Can you work these out from the model? Positions are in its coordinate system, mm. Face numbers are marked on the shaded views. A direction names the side the tool comes from. Coordinates: 2 decimals unless noted, no trailing zeros. Write each loop counter-clockwise with the first axis right and the second up, starting at its lowest first coordinate (ties: lowest second). Pieces come first, ordered by that corner, then holes.
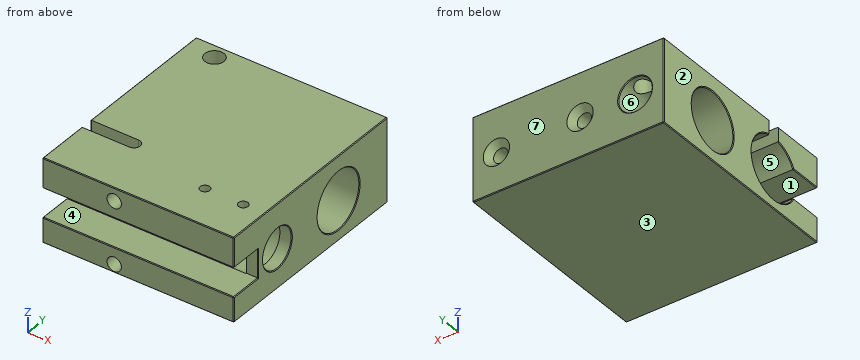
```python
from build123d import *

# Parameters (mm, degrees)
ESQUISSE1_W                   = 80
ESQUISSE1_H                   = 88
BASE_EXTRUSION_DEPTH          = 35
ESQUISSE4_R                   = 12
BOSS_EXTRU_2_DEPTH            = 80
ESQUISSE5_R                   = 12
ENL_V_MAT_EXTRU_1_DEPTH       = 145
ESQUISSE6_W                   = 12
ESQUISSE6_H                   = 14
ENL_V_MAT_EXTRU_2_DEPTH       = 145
ESQUISSE12_R                  = 12.75
ENL_V_MAT_EXTRU_4_DEPTH       = 75
ESQUISSE13_R                  = 8.25
ENL_V_MAT_EXTRU_5_DEPTH       = 94.733665244
ESQUISSE17_W                  = 20
ESQUISSE17_H                  = 5.2
ENL_V_MAT_EXTRU_9_DEPTH       = 10
ESQUISSE18_R                  = 2.6
ENL_V_MAT_EXTRU_10_DEPTH      = 10
ESQUISSE20_R                  = 2.25
ENL_V_MAT_EXTRU_12_DEPTH      = 14
ESQUISSE21_R                  = 3
ENL_V_MAT_EXTRU_13_DEPTH      = 10
CHANFREIN9_SIZE               = 1.154700538
CHANFREIN9_SIZE2              = 2
CHANFREIN20_SIZE              = 1.154700538
CHANFREIN20_SIZE2             = 2
ESQUISSE22_R                  = 2
ENL_V_MAT_EXTRU_15_DEPTH      = 5.5
ESQUISSE24_R                  = 7
ENL_V_MAT_EXTRU_23_DEPTH      = 25
ENL_V_MAT_EXTRU_24_REACH      = 71
ENL_V_MAT_EXTRU_24_END_RADIUS = 7
ESQUISSE25_R                  = 4
ESQUISSE26_R                  = 2.5
ENL_V_MAT_EXTRU_25_DEPTH      = 15
ESQUISSE28_R                  = 3
ENL_V_MAT_EXTRU_26_DEPTH      = 12
CHANFREIN27_SIZE              = 2.5
CHANFREIN29_SIZE              = 0.3


with BuildPart() as part:
    # Esquisse1 → Base-Extrusion (new body)
    with BuildSketch(Plane.XY):
        Rectangle(ESQUISSE1_W, ESQUISSE1_H)
    extrude(amount=BASE_EXTRUSION_DEPTH)

    # Esquisse4 → Boss.-Extru.2 (add, through all)
    with BuildSketch(Plane.ZY.offset(40)):
        with Locations((16.5, 16)):
            Circle(ESQUISSE4_R)
    extrude(amount=-BOSS_EXTRU_2_DEPTH)

    # Esquisse5 → Enlèv. mat.-Extru.1 (cut)
    with BuildSketch(Plane.ZY.offset(40)):
        with Locations((16.5, 16)):
            Circle(ESQUISSE5_R)
    extrude(amount=-ENL_V_MAT_EXTRU_1_DEPTH, mode=Mode.SUBTRACT)

    # Esquisse6 → Enlèv. mat.-Extru.2 (cut)
    with BuildSketch(Plane(origin=(40, 0, 0), x_dir=(0, 0, -1), z_dir=(1, 0, 0))):
        with Locations((-16.5, -37)):
            Rectangle(ESQUISSE6_W, ESQUISSE6_H)
    extrude(amount=-ENL_V_MAT_EXTRU_2_DEPTH, mode=Mode.SUBTRACT)

    # Esquisse12 → Enlèv. mat.-Extru.4 (cut)
    with BuildSketch(Plane.ZY.offset(40)):
        with Locations((16.5, -19)):
            Circle(ESQUISSE12_R)
    extrude(amount=-ENL_V_MAT_EXTRU_4_DEPTH, mode=Mode.SUBTRACT)

    # Esquisse13 → Enlèv. mat.-Extru.5 (cut, through all)
    with BuildSketch(Plane.ZY.offset(-35)):
        with Locations((16.5, -19)):
            Circle(ESQUISSE13_R)
    extrude(amount=-ENL_V_MAT_EXTRU_5_DEPTH, mode=Mode.SUBTRACT)

    # Esquisse17 → Enlèv. mat.-Extru.9 (cut)
    with BuildSketch(Plane.XY.offset(35)):
        with Locations((-30, -19)):
            Rectangle(ESQUISSE17_W, ESQUISSE17_H)
    extrude(amount=-ENL_V_MAT_EXTRU_9_DEPTH, mode=Mode.SUBTRACT)

    # Esquisse18 → Enlèv. mat.-Extru.10 (cut)
    with BuildSketch(Plane.XY.offset(35)):
        with Locations((-20, -19)):
            Circle(ESQUISSE18_R)
    extrude(amount=-ENL_V_MAT_EXTRU_10_DEPTH, mode=Mode.SUBTRACT)

    # Esquisse20 → Enlèv. mat.-Extru.12 (cut)
    with BuildSketch(Plane.XZ.offset(44)):
        with Locations(Location((-10, 29.5, 0), (0, 0, 270))):
            Circle(ESQUISSE20_R)
        with Locations(Location((-10, 3.5, 0), (0, 0, 90))):
            Circle(ESQUISSE20_R)
    extrude(amount=-ENL_V_MAT_EXTRU_12_DEPTH, mode=Mode.SUBTRACT)

    # Esquisse21 → Enlèv. mat.-Extru.13 (cut)
    with BuildSketch(Plane.XZ.offset(44)):
        with Locations(Location((-10, 3.5, 0), (0, 0, 270))):
            Circle(ESQUISSE21_R)
        with Locations(Location((-10, 29.5, 0), (0, 0, 90))):
            Circle(ESQUISSE21_R)
    extrude(amount=-ENL_V_MAT_EXTRU_13_DEPTH, mode=Mode.SUBTRACT)

    # Chanfrein9
    chanfrein9_edges = [part.edges().sort_by_distance(p)[0] for p in [
        (-10, -30, 1.25),
    ]]
    chanfrein9_side = [part.faces().sort_by_distance(p)[0] for p in [
        (-10, -32, 1.25),
    ]]
    chamfer(chanfrein9_edges, length=CHANFREIN9_SIZE, length2=CHANFREIN9_SIZE2, reference=chanfrein9_side[0])

    # Chanfrein20
    chanfrein20_edges = [part.edges().sort_by_distance(p)[0] for p in [
        (-10, -30, 31.75),
    ]]
    chanfrein20_side = [part.faces().sort_by_distance(p)[0] for p in [
        (-10, -32, 31.75),
    ]]
    chamfer(chanfrein20_edges, length=CHANFREIN20_SIZE, length2=CHANFREIN20_SIZE2, reference=chanfrein20_side[0])

    # Esquisse22 → Enlèv. mat.-Extru.15 (cut)
    with BuildSketch(Plane.XY.offset(35)):
        with Locations((31, -26.25)):
            Circle(ESQUISSE22_R)
        with Locations((15, -26.25)):
            Circle(ESQUISSE22_R)
    extrude(amount=-ENL_V_MAT_EXTRU_15_DEPTH, mode=Mode.SUBTRACT)

    # Esquisse24 → Enlèv. mat.-Extru.23 (cut)
    with BuildSketch(Plane(origin=(0, 44, 0), x_dir=(-1, 0, 0), z_dir=(0, 1, 0))):
        with Locations((28, 16.5)):
            Circle(ESQUISSE24_R)
    extrude(amount=-ENL_V_MAT_EXTRU_23_DEPTH, mode=Mode.SUBTRACT)

    # Enlèv. mat.-Extru.24: up to this cylinder (the profile starts outside it)
    enl_v_mat_extru_24_end = Plane(origin=(-28, 38, 16.5), z_dir=(0, 1, 0)) * Cylinder(ENL_V_MAT_EXTRU_24_END_RADIUS, 157, mode=Mode.PRIVATE)
    # Esquisse25 → Enlèv. mat.-Extru.24 (cut, up to the surface)
    with BuildSketch(Plane.XY.offset(35), mode=Mode.PRIVATE) as enl_v_mat_extru_24_sk1:
        with Locations((-28, 38)):
            Circle(ESQUISSE25_R)
    enl_v_mat_extru_24_tool1 = extrude(enl_v_mat_extru_24_sk1.sketch, amount=-ENL_V_MAT_EXTRU_24_REACH, mode=Mode.PRIVATE) - enl_v_mat_extru_24_end
    add(enl_v_mat_extru_24_tool1.solids().sort_by_distance((-28, 38, 35))[0], mode=Mode.SUBTRACT)

    # Esquisse26 → Enlèv. mat.-Extru.25 (cut)
    with BuildSketch(Plane(origin=(0, 44, 0), x_dir=(-1, 0, 0), z_dir=(0, 1, 0))):
        with Locations((-30, 16.5)):
            Circle(ESQUISSE26_R)
        with Locations((5, 16.5)):
            Circle(ESQUISSE26_R)
    extrude(amount=-ENL_V_MAT_EXTRU_25_DEPTH, mode=Mode.SUBTRACT)

    # Esquisse28 → Enlèv. mat.-Extru.26 (cut)
    with BuildSketch(Plane(origin=(0, 44, 0), x_dir=(-1, 0, 0), z_dir=(0, 1, 0))):
        with Locations((-30, 16.5)):
            Circle(ESQUISSE28_R)
        with Locations((5, 16.5)):
            Circle(ESQUISSE28_R)
    extrude(amount=-ENL_V_MAT_EXTRU_26_DEPTH, mode=Mode.SUBTRACT)

    # Chanfrein27
    chanfrein27_edges = [part.edges().sort_by_distance(p)[0] for p in [
        (33, 44, 16.5),
        (-2, 44, 16.5),
    ]]
    chamfer(chanfrein27_edges, length=CHANFREIN27_SIZE)

    # Chanfrein29
    chanfrein29_edges = [part.edges().sort_by_distance(p)[0] for p in [
        (40, 0, 35),
        (-21, 44, 16.5),
        (0, 44, 35),
        (40, 16, 4.5),
        (-40, 16, 4.5),
        (40, -44, 5.25),
        (-40, -44, 5.25),
        (0, -44, 10.5),
        (0, -44, 22.5),
        (40, -37, 22.5),
        (40, -30, 16.5),
        (40, -37, 10.5),
        (-40, -37.125, 22.5),
        (-40, 13.8, 35),
        (-40, -37.125, 10.5),
        (0, 44, 0),
        (-40, -26.64591319, 26.703063829),
        (40, 0, 0),
        (0, -44, 0),
        (40, -19, 8.25),
        (-40, 0, 0),
        (-40, -8.796936171, 8.85408681),
        (-40, -32.8, 35),
        (-40, -16.4, 31.991043583),
        (0, -44, 35),
        (-40, 44, 17.5),
        (40, 44, 17.5),
        (40, -44, 28.75),
        (-40, -44, 28.75),
    ]]
    chamfer(chanfrein29_edges, length=CHANFREIN29_SIZE)


solid = part.part
```
1. I'm going to push flat-ended pins straight in: P1, Ø4, axis at x = -10, z = 3.5, coming from the -Y side; P2, Ø1.4, axis at x = 37.5, z = 15, coming from the -Y side; P3, Ø1.8, axis at x = 29, z = 15, coming from the +Y side. Where does each tip first touch, or does it pass through?
2. If we section it at A-A, the plane y = -19: List the corners of the cut face in (x, z) for me.
3. If we section it at B-B, the plane x = -5: List the corners of the cut face in (y, z) for me.
4. We'd pull the mould along Z, two halves only. Please class the marked faces 1, 2, 3 and 4: released by +Z, released by -Z, zero draft, split by the parting line, or undercut.
5. Which directions (+Z, -Z, +X, -X, +Y, -Y) give clear straight access to the entire face, cutting with the end or side of a thin tool? Please do the marked faces 5, 6 and 7.
6. If we section it at C-C, the plane y = 38: List the corners of the cut face in (x, z) for me, plus the area to 3 significant figures.
7. If I drill on L1, parallel to Y at x = 37.6, z = 16.5; L2, parallel to Y at x = -28, z = 30; L3, parallel to Z at x = -5, y = 31.35, over which ranges is the centre line in solid material (lowest first)?
8. If we section it at D-D, the plane x = 15: List the corners of the cut face in (y, z) for me.
Answers:
1. P1: stops at y = -31.01
1. P2: stops at y = -30
1. P3: stops at y = 32
2. outline: (-40, 0.3) - (-39.7, 0) - (39.7, 0) - (40, 0.3) - (40, 7.95) - (39.7, 8.25) - (35, 8.25) - (35, 3.75) - (-39.7, 3.75) - (-40, 3.45) - close; (-17.4, 29.25) - (35, 29.25) - (35, 24.75) - (39.7, 24.75) - (40, 25.05) - (40, 34.7) - (39.7, 35) - (-17.4, 35) - close
3. outline: (-44, 0.3) - (-43.7, 0) - (43.7, 0) - (44, 0.3) - (44, 11) - (41.5, 13.5) - (32, 13.5) - (32, 14) - (29, 14) - (29, 19) - (32, 19) - (32, 19.5) - (41.5, 19.5) - (44, 22) - (44, 34.7) - (43.7, 35) - (-43.7, 35) - (-44, 34.7) - (-44, 22.8) - (-43.7, 22.5) - (-30.25, 22.5) arc R12.75 cw (long way) to (-30.25, 10.5) - (-43.7, 10.5) - (-44, 10.2) - close; hole circle Ø24 at (16, 16.5)
4. face 1: undercut
4. face 2: zero draft
4. face 3: released by -Z
4. face 4: undercut
5. face 5: -X
5. face 6: +Y
5. face 7: +Z, -Z, +X, -X, +Y
6. outline: (-40, 0.3) - (-39.7, 0) - (39.7, 0) - (40, 0.3) - (40, 34.7) - (39.7, 35) - (-24, 35) - (-24, 22.24) arc R7 cw (long way) to (-32, 22.24) - (-32, 35) - (-39.7, 35) - (-40, 34.7) - close; hole circle Ø6 at (-5, 16.5); hole circle Ø6 at (30, 16.5)
6. area: 2,490 mm2
7. L1: y = -30 to -27.25, -10.75 to 4, 28 to 44
7. L2: y = -44 to -21.6, -16.4 to 34, 42 to 44
7. L3: z = 0 to 14, 19 to 35
8. outline: (-44, 0.3) - (-43.7, 0) - (43.7, 0) - (44, 0.3) - (44, 34.7) - (43.7, 35) - (-24.25, 35) - (-24.25, 29.5) - (-28.25, 29.5) - (-28.25, 35) - (-43.7, 35) - (-44, 34.7) - (-44, 22.8) - (-43.7, 22.5) - (-30.25, 22.5) arc R12.75 cw (long way) to (-30.25, 10.5) - (-43.7, 10.5) - (-44, 10.2) - close; hole circle Ø24 at (16, 16.5)
